The listing builds one solid part. Answer for the finished solid, in the listing's coordinates (mm). A direction names the side the tool comes from. Give positions to 0.01 mm unless a question says otherwise; leave off trailing zeros. Write each loop counter-clockwise with the first axis right and the second up, starting at its lowest first coordinate (ties: lowest second). Pieces come first, ordered by that corner, then holes. Notation, with made-up numbers: (3.25, -13.75) - (26.25, -13.75) arc R20 cw to (26.25, -5.75) - close; hole circle Ø9 at (6, 52.25). An arc over 180 degrees is marked (long way). One line per question, with ' | ' between items. Start each with the question number.
1. Given P1, Ø10, axis at x = 21.5, y = 19.5, coming from the -Z side, flat-ended and moving along its own axis, determine where the tip first touches the part or whether it passes through.
2. Find the intervals of material crossed by L1, parallel to Y at x = 34, z = -6.5, in increasing order. Write a range as from..to.
3. A cutting plane is placed at A-A (z = -14.5). Determine the outline of the cut face in (x, y), then the cut area to 3 significant figures.
4. The mould has two halves that part along Y. Classify faces 4 (the face through (33, 1.129, -13)), 5 (the face through (5.34, 51, -13)), 6 (the face through (3, 49.97, -13)), 7 (the face through (4, 0, -13)): +Y half, -Y half, draft (parallel to the pull), parting line (faces both ways), or undercut.
5. For faces 1 (the face through (36.041, 0.6, -12.5)), 2 (the face through (27.806, 52, -13)), 3 (the face through (3, 2.032, -13)), determine the directions among +Z, -Z, +X, -X, +Y, -Y from which every point of the face is accessible in a straight line to the end or side of a thin tool.
```python
from build123d import *

# Parameters (mm, degrees)
F0_W     = 36.041372
F0_H     = 52.817661
F0_R     = 6.880185
F1_DEPTH = 0.0254
F2_W     = 6.246955
F2_H     = 1.12941
F2_W_2   = 6.467774
F2_H_2   = 2.031927
F2_W_3   = 8.2353
F2_H_3   = 1.951657
F2_W_4   = 5.340438
F2_H_4   = 2.847552
F3_DEPTH = 25.4


with BuildPart() as f1:
    # F0 (on Top) → F1 (new body)
    with BuildSketch(Plane.XY):
        with Locations((18.020686, 26.408831)):
            Rectangle(F0_W, F0_H)
        with Locations((18.543148, 12.65093)):
            Circle(F0_R, mode=Mode.SUBTRACT)
    extrude(amount=F1_DEPTH)

    # F2 (on face) → F3 (join)
    with BuildSketch(Plane.XY.offset(0.0254)):
        with Locations((32.917894, 0.564705)):
            Rectangle(F2_W, F2_H)
        with Locations((3.233887, 1.015964)):
            Rectangle(F2_W_2, F2_H_2)
        with Locations((31.923722, 51.841832)):
            Rectangle(F2_W_3, F2_H_3)
        with Locations((2.670219, 51.393885)):
            Rectangle(F2_W_4, F2_H_4)
    extrude(amount=-F3_DEPTH)


solid = f1.part
```
Determined:
1) P1: z = 0
2) L1: 0..1.13, 50.87..52.82
3) outline: (0, 0) - (6.47, 0) - (6.47, 2.03) - (0, 2.03) - close; (0, 49.97) - (5.34, 49.97) - (5.34, 52.82) - (0, 52.82) - close; (27.81, 50.87) - (36.04, 50.87) - (36.04, 52.82) - (27.81, 52.82) - close; (29.79, 0) - (36.04, 0) - (36.04, 1.13) - (29.79, 1.13) - close | area: 51.5 mm2
4) face 4: undercut | face 5: draft | face 6: undercut | face 7: -Y half
5) face 1: +Z, -Z, +X, +Y, -Y | face 2: -Z, +Y, -Y | face 3: -Z, +X, -X
